```python
from build123d import *

# Parameters (mm, degrees)
SKETCH1_R           = 8
BOSS_EXTRUDE1_DEPTH = 7
CUT_EXTRUDE1_DEPTH  = 10
SKETCH3_R           = 3.1
CUT_EXTRUDE2_DEPTH  = 6
FILLET1_R           = 0.5
FILLET2_R           = 1
FILLET3_R           = 1
FILLET5_R           = 1
FILLET6_R           = 0.5
FILLET7_R           = 1


with BuildPart() as part:
    # Sketch1 → Boss-Extrude1 (new body)
    with BuildSketch(Plane(origin=(0, 0, 0), x_dir=(1, 0, 0), z_dir=(0, 1, 0))):
        with BuildLine():
            Line((-37.5, -15), (37.5, -15))
            ThreePointArc((37.5, -15), (44.571067812, -12.071067812), (47.5, -5))
            Line((47.5, -5), (47.5, 5))
            ThreePointArc((47.5, 5), (44.571067812, 12.071067812), (37.5, 15))
            Line((37.5, 15), (-37.5, 15))
            ThreePointArc((-37.5, 15), (-44.571067812, 12.071067812), (-47.5, 5))
            Line((-47.5, 5), (-47.5, -5))
            ThreePointArc((-47.5, -5), (-44.571067812, -12.071067812), (-37.5, -15))
        make_face()
        with Locations(Location((0, 0, 0), (0, 0, 270))):
            Circle(SKETCH1_R, mode=Mode.SUBTRACT)
    extrude(amount=BOSS_EXTRUDE1_DEPTH)

    # Sketch2 → Cut-Extrude1 (cut)
    with BuildSketch(Plane(origin=(0, 7, 0), x_dir=(1, 0, 0), z_dir=(0, 1, 0))):
        with BuildLine():
            Line((-19.25, 0), (-19.25, 15))
            Line((-19.25, 15), (-43.85, 15))
            Line((-43.85, 15), (-43.85, 0))
            ThreePointArc((-43.85, 0), (-31.55, -12.3), (-19.25, 0))
        make_face()
    cut_extrude1 = extrude(amount=-CUT_EXTRUDE1_DEPTH, mode=Mode.SUBTRACT)

    # Sketch3 → Cut-Extrude2 (cut)
    with BuildSketch(Plane.ZY.offset(19.25)):
        with Locations((-11.34873736, 3.5)):
            Circle(SKETCH3_R)
    cut_extrude2 = extrude(amount=-CUT_EXTRUDE2_DEPTH, mode=Mode.SUBTRACT)

    # Fillet1
    # the kernel refuses this fillet: 0.5 mm, written as the material it takes off along each edge
    with BuildSketch(Plane(origin=(-19.25, 3.5, -11.34873736), x_dir=(0, 0, 1), z_dir=(0, -1, 0))) as fillet1_piece_1:
        with BuildLine():
            CenterArc((3.1 + FILLET1_R, -FILLET1_R), FILLET1_R, 90, 90)
            Line((3.1, -FILLET1_R), (3.1, 0))
            Line((3.1, 0), (3.1 + FILLET1_R, 0))
        make_face()
    revolve(axis=Axis((-19.25, 3.5, -11.34873736), (-1, 0, 0)), mode=Mode.SUBTRACT)

    # Fillet2
    fillet2_edges = [part.edges().sort_by_distance(p)[0] for p in [
        (-43.85, 3.5, -12.725121358),
    ]]
    fillet(fillet2_edges, radius=FILLET2_R)

    # Fillet3
    # the kernel refuses this fillet: 1 mm, written as the material it takes off along each edge
    with BuildSketch(Plane(origin=(-19.25, 9.5, -15), x_dir=(0, 0, 1), z_dir=(0, -1, 0))) as fillet3_piece_1:
        with BuildLine():
            CenterArc((FILLET3_R, -FILLET3_R), FILLET3_R, 90, 90)
            Line((0, -FILLET3_R), (-FILLET3_R * 0.02, -FILLET3_R))
            Line((-FILLET3_R * 0.02, -FILLET3_R), (-FILLET3_R * 0.02, FILLET3_R * 0.02))
            Line((-FILLET3_R * 0.02, FILLET3_R * 0.02), (FILLET3_R, FILLET3_R * 0.02))
            Line((FILLET3_R, FILLET3_R * 0.02), (FILLET3_R, 0))
        make_face()
    extrude(amount=12, mode=Mode.SUBTRACT)

    # Mirror5: Cut-Extrude1, Cut-Extrude2 across plane
    add(cut_extrude1.mirror(Plane.ZY), mode=Mode.SUBTRACT)
    add(cut_extrude2.mirror(Plane.ZY), mode=Mode.SUBTRACT)

    # Fillet5
    fillet5_edges = [part.edges().sort_by_distance(p)[0] for p in [
        (43.85, 3.5, -12.725121358),
    ]]
    fillet(fillet5_edges, radius=FILLET5_R)

    # Fillet6
    # the kernel refuses this fillet: 0.5 mm, written as the material it takes off along each edge
    with BuildSketch(Plane(origin=(19.25, 3.5, -11.34873736), x_dir=(0, 0, 1), z_dir=(0, -1, 0))) as fillet6_piece_1:
        with BuildLine():
            CenterArc((3.1 + FILLET6_R, FILLET6_R), FILLET6_R, 180, 90)
            Line((3.1, FILLET6_R), (3.1, 0))
            Line((3.1, 0), (3.1 + FILLET6_R, 0))
        make_face()
    revolve(axis=Axis((19.25, 3.5, -11.34873736), (-1, 0, 0)), mode=Mode.SUBTRACT)

    # Fillet7
    # the kernel refuses this fillet: 1 mm, written as the material it takes off along each edge
    with BuildSketch(Plane(origin=(19.25, 9.5, -15), x_dir=(-1, 0, 0), z_dir=(0, -1, 0))) as fillet7_piece_1:
        with BuildLine():
            CenterArc((FILLET7_R, -FILLET7_R), FILLET7_R, 90, 90)
            Line((0, -FILLET7_R), (-FILLET7_R * 0.02, -FILLET7_R))
            Line((-FILLET7_R * 0.02, -FILLET7_R), (-FILLET7_R * 0.02, FILLET7_R * 0.02))
            Line((-FILLET7_R * 0.02, FILLET7_R * 0.02), (FILLET7_R, FILLET7_R * 0.02))
            Line((FILLET7_R, FILLET7_R * 0.02), (FILLET7_R, 0))
        make_face()
    extrude(amount=12, mode=Mode.SUBTRACT)


solid = part.part
```
Check sheet for the modelled part. Datum: model origin and axes. Units: mm. A direction names the side the tool comes from. Coordinates: 2 decimals unless noted, no trailing zeros. Write each loop counter-clockwise with the first axis right and the second up, starting at its lowest first coordinate (ties: lowest second). Pieces come first, ordered by that corner, then holes. Notation, with made-up numbers: M -10.75,56.25 L 27.25,56.25 A9 cw 27.25,68.25 Z; hole C 78.5,19.25 d10. An arc over 180 degrees is marked long. Write item = value, one per line. Start each with the question number.
1. Thickness scan on probe 1 along X at (y, z) = (3, 1.5); probe 2 along X at (y, z) = (3, -7); probe 3 along X at (y, z) = (6, -8.5). Record the ranges inside material, lowest first.
2. Tool access check on faces 5 (the flat face through (-19.25, 4, -4)), 6 (the cylindrical face through (-16.038, 0.474, -12.021)), 7 (the cylindrical face through (-44.65, 3.45, 11.99)). Record the directions out of +Z, -Z, +X, -X, +Y, -Y that give a thin tool (end or side, any length) a straight path to the whole face; none if there is none.
3. Sectioned sample at D-D (x = 21). Record the cut outline in (y, z), then the cut area to 3 significant figures.
4. Sectioned sample at C-C (x = 31.55). Record the cut outline in (y, z).
5. Go/stop test with flat-tipped pins: pin 1 (1.2 mm diameter, centred on y = 0.5, z = -13, fed in from +X); pin 2 (4 mm diameter, centred on x = 24, y = 3, fed in from -Z); pin 3 (2 mm diameter, centred on y = 4, z = 8.5, fed in from +X). Record where each tip stops, or that it passes through.
6. Sectioned sample at A-A (x = 0). Record the cut outline in (y, z), then the cut area to 3 significant figures.
7. Mould release check, pull along Y, two halves, no side actions. Record for faces 1 (the flat face through (-1, 0, 10)), 2 (the flat face through (19.25, 4, -4)), 3 (the cylindrical face through (16.038, 0.474, -12.021)), 4 (the flat face through (-13.25, 4, -11)): pulls with the +Y half, pulls with the -Y half, needs draft (parallel to the pull), parting line crosses it, or undercut.
The answers:
q1.probe_1 = -47.5 to -43.76, -19.34 to -7.86, 7.86 to 19.34, 43.76 to 47.5
q1.probe_2 = -47.3 to -43.85, -19.25 to -3.87, 3.87 to 19.25, 43.85 to 47.3
q1.probe_3 = -46.87 to -43.85, -19.25 to 19.25, 43.85 to 46.87
q2.face_5 = -Z, +Y, -Y
q2.face_6 = none
q2.face_7 = +Z, -X, +Y, -Y
q3.outline = M 0,6.32 L 7,6.32 L 7,15 L 0,15 Z
q3.area = 60.7 mm²
q4.outline = M 0,12.3 L 7,12.3 L 7,15 L 0,15 Z
q5.pin_1 = 19.25
q5.pin_2 = 7.75
q5.pin_3 = 47.18
q6.outline = M 0,-15 L 7,-15 L 7,-8 L 0,-8 Z; M 0,8 L 7,8 L 7,15 L 0,15 Z
q6.area = 98.0 mm²
q7.face_1 = pulls with the -Y half
q7.face_2 = needs draft
q7.face_3 = undercut
q7.face_4 = undercut
